Verification items for this drawing (mm, ordinates from the low corner). A direction names the side the tool comes from. Coordinates: 2 decimals unless noted, no trailing zeros. Order: outer loops, then holes, each group sorted by start corner. A loop starts at its lowest first (then second) coordinate and runs counter-clockwise, first axis right, second up. Notation, with made-up numbers: (85, 60.5) -> (127, 60.5) arc R31 cw to (127, 85.5) -> close; hole circle Ø6 at (78.5, 82.5). An arc over 180 degrees is marked (long way). Write item = value, one per line. Start each with the question number.
1. Set-up check for the marked faces 4, 5 and 6: record each of +Z, -Z, +X, -X, +Y, -Y from which the full face is reachable in a straight line by a thin tool's end or side.
2. Thickness scan on line 1 along Y through (x, z) = (84.5, 56); line 2 along Z through (x, y) = (59, 2); line 3 along Y through (x, z) = (21, 40.5). Record the ranges inside material, lowest first. Write a range as from..to.
3. Cross-section at A-A on x = 43. Record the cut outline in (y, z), plus the area to 3 significant figures.
4. Release check for a two-part mould opening along X. For the marked faces 1, 2 and 3 record: +X half, -X half, draft (parallel to the pull), parting line (faces both ways), or undercut.
5. Cross-section at C-C on y = 5.5. Record the cut outline in (x, z).
6. Cross-section at B-B on z = 58. Record the cut outline in (x, y).
7. Go/stop test with flat-tipped pins: P1, Ø4, axis at x = 71, y = 16.5, coming from the -Z side; P2, Ø1.2, axis at y = 31, z = 27.5, coming from the -X side; P3, Ø4.5, axis at y = 32, z = 31, coming from the +X side; P4, Ø3, axis at x = 95.5, z = 55, coming from the +Y side. Record where each tip stops, or that it passes through.
8. Cross-section at D-D on x = 18. Record the cut outline in (y, z), plus the area to 3 significant figures.
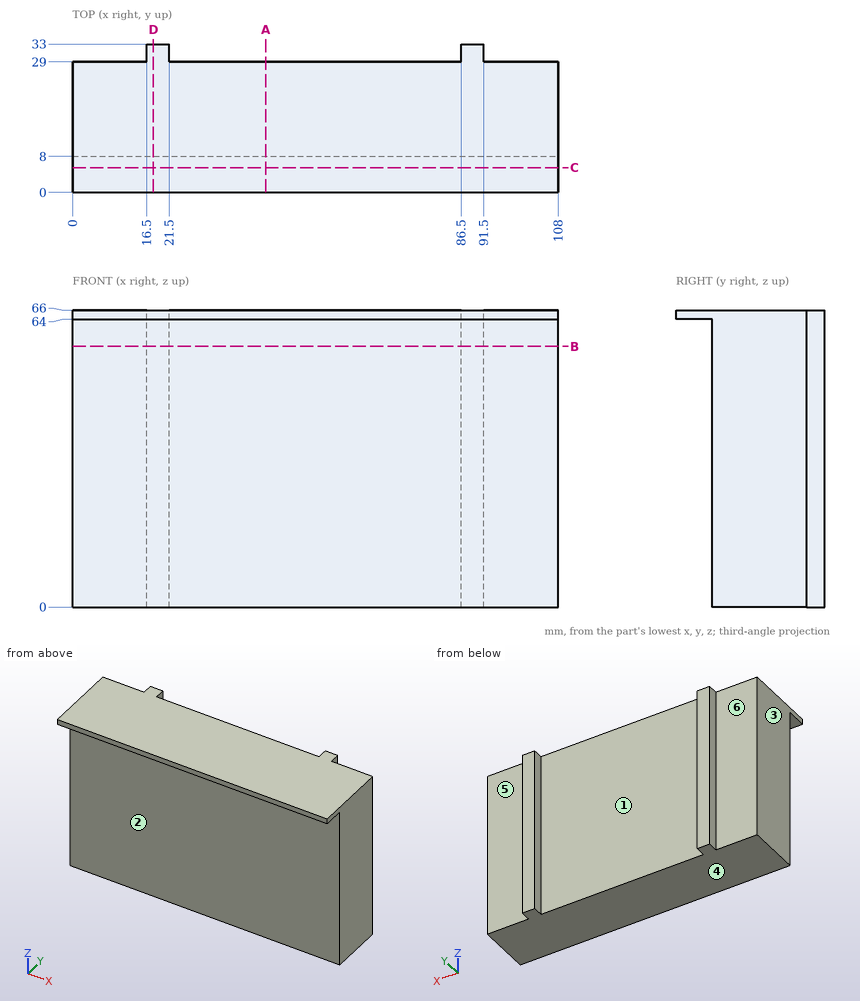
Worked out:
q1.face_4 = -Z, +X, -X, +Y, -Y
q1.face_5 = +Z, -Z, +X, +Y
q1.face_6 = +Z, -Z, -X, +Y
q2.line_1 = 8..29
q2.line_2 = 64..66
q2.line_3 = 8..33
q3.outline = (0, 64) -> (8, 64) -> (8, 0) -> (29, 0) -> (29, 66) -> (0, 66) -> close
q3.area = 1,400 mm²
q4.face_1 = undercut
q4.face_2 = draft
q4.face_3 = -X half
q5.outline = (0, 64) -> (108, 64) -> (108, 66) -> (0, 66) -> close
q6.outline = (0, 8) -> (108, 8) -> (108, 29) -> (91.5, 29) -> (91.5, 33) -> (86.5, 33) -> (86.5, 29) -> (21.5, 29) -> (21.5, 33) -> (16.5, 33) -> (16.5, 29) -> (0, 29) -> close
q7.P1 = 0
q7.P2 = 16.5
q7.P3 = 91.5
q7.P4 = 29
q8.outline = (0, 64) -> (8, 64) -> (8, 0) -> (33, 0) -> (33, 66) -> (0, 66) -> close
q8.area = 1,670 mm²
